Verification items for the finished model (mm, model axes). Round coordinates to 2 decimals unless told otherwise and drop trailing zeros. Order: outer loops, then holes, each group sorted by start corner. A loop starts at its lowest first (then second) coordinate and runs counter-clockwise, first axis right, second up. Notation, with made-up numbers: M 22.25,48.5 L 71.25,48.5 A36 ccw 71.25,84.5 Z; hole C -28.75,47.25 d7. An arc over 180 degrees is marked long. Use CSV: the item, a comma, the result in double quotes. Start each with the question number.
Q1. Gauge pin test, flat ends, axial feed: pin 1 Ø1.6 at (y, z) = (1, -34) entering from -X; pin 2 Ø1.1 at (y, z) = (2, -222) entering from +X; pin 3 Ø1 at (y, z) = (2, -64) entering from -X. Record the tip position at first contact, or that the pin passes through.
Q2. Sectioned sample at A-A (y = 0.75). State how many separate pieces and enclosed holes the cut face has, and give its area (3 significant figures).
Q3. Sectioned sample at B-B (z = -500). Enter the section's corners in (x, y).
Q4. Scan lines: line 1 (X direction, y = 0.95, z = -95); line 2 (X direction, y = 0.5, z = -28); line 3 (X direction, y = 1.1, z = -175). Record each from-to range of solid material in increasing order.
```python
from build123d import *

# Parameters (mm, degrees)
SALIENTE_EXTRUIR1_DEPTH = 3.2
CROQUIS3_R              = 2.05
CORTAR_EXTRUIR2_DEPTH   = 3.2
CORTAR_EXTRUIR3_DEPTH   = 3.2
CORTAR_EXTRUIR4_DEPTH   = 3.2
REDONDEO1_R             = 3
CROQUIS6_R              = 1.55
CORTAR_EXTRUIR5_DEPTH   = 3.2
CROQUIS7_W              = 3
CROQUIS7_H              = 0.2
CORTAR_EXTRUIR6_DEPTH   = 3.2


with BuildPart() as part:
    # Croquis1 → Saliente-Extruir1 (new body)
    with BuildSketch(Plane(origin=(0, 0, 0), x_dir=(1, 0, 0), z_dir=(0, 1, 0))):
        Polygon((7, 66.1), (10, 66.1), (10, 62.9), (7, 62.9), (7, 61.5), (3, 61.5), (3, 62.9), (0, 62.9), (0, 57), (-3, 57), (-3, 51), (0, 51), (0, 0), (165, 0), (165, 1.5), (168, 1.5), (168, 7.5), (165, 7.5), (165, 13.4), (162, 13.4), (162, 12), (158, 12), (158, 13.4), (155, 13.4), (155, 16.6), (158, 16.6), (158, 18), (162, 18), (162, 16.6), (165, 16.6), (165, 22.5), (168, 22.5), (168, 28.5), (165, 28.5), (165, 570), (30, 570), (30, 566.9), (21.6, 566.9), (21.6, 563.9), (23, 563.9), (23, 559.9), (21.6, 559.9), (21.6, 556.9), (18.4, 556.9), (18.4, 559.9), (17, 559.9), (17, 563.9), (18.4, 563.9), (18.4, 566.9), (10, 566.9), (10, 570), (0, 570), (0, 543), (-3, 543), (-3, 537), (0, 537), (0, 531.1), (3, 531.1), (3, 532.5), (7, 532.5), (7, 531.1), (10, 531.1), (10, 527.9), (7, 527.9), (7, 526.5), (3, 526.5), (3, 527.9), (0, 527.9), (0, 522), (-3, 522), (-3, 516), (0, 516), (0, 388), (-3, 388), (-3, 382), (0, 382), (0, 376.1), (3, 376.1), (3, 377.5), (7, 377.5), (7, 376.1), (10, 376.1), (10, 372.9), (7, 372.9), (7, 371.5), (3, 371.5), (3, 372.9), (0, 372.9), (0, 367), (-3, 367), (-3, 361), (0, 361), (0, 233), (-3, 233), (-3, 227), (0, 227), (0, 221.1), (3, 221.1), (3, 222.5), (7, 222.5), (7, 221.1), (10, 221.1), (10, 217.9), (7, 217.9), (7, 216.5), (3, 216.5), (3, 217.9), (0, 217.9), (0, 212), (-3, 212), (-3, 206), (0, 206), (0, 78), (-3, 78), (-3, 72), (0, 72), (0, 66.1), (3, 66.1), (3, 67.5), (7, 67.5), align=None)
    extrude(amount=SALIENTE_EXTRUIR1_DEPTH)

    # Croquis3 → Cortar-Extruir2 (cut)
    with BuildSketch(Plane(origin=(0, 3.2, 0), x_dir=(1, 0, 0), z_dir=(0, 1, 0))):
        with Locations((40, 80)):
            Circle(CROQUIS3_R)
        with Locations((90, 80)):
            Circle(CROQUIS3_R)
        with Locations((40, 230)):
            Circle(CROQUIS3_R)
    extrude(amount=-CORTAR_EXTRUIR2_DEPTH, mode=Mode.SUBTRACT)

    # Croquis4 → Cortar-Extruir3 (cut)
    with BuildSketch(Plane.XZ):
        with BuildLine():
            Line((143, -30.5), (129, -30.5))
            ThreePointArc((129, -30.5), (127.585786438, -31.085786438), (127, -32.5))
            Line((127, -32.5), (127, -38.5))
            ThreePointArc((127, -38.5), (127.585786438, -39.914213562), (129, -40.5))
            Line((129, -40.5), (143, -40.5))
            ThreePointArc((143, -40.5), (144.414213562, -39.914213562), (145, -38.5))
            Line((145, -38.5), (145, -32.5))
            ThreePointArc((145, -32.5), (144.414213562, -31.085786438), (143, -30.5))
        make_face()
    extrude(amount=-CORTAR_EXTRUIR3_DEPTH, mode=Mode.SUBTRACT)

    # Croquis5 → Cortar-Extruir4 (cut)
    with BuildSketch(Plane.XZ):
        with BuildLine():
            Line((35, -570), (165, -570))
            Line((165, -570), (165, -31.5))
            ThreePointArc((165, -31.5), (70.982951471, -293.744955787), (35, -570))
        make_face()
    extrude(amount=-CORTAR_EXTRUIR4_DEPTH, mode=Mode.SUBTRACT)

    # Redondeo1
    redondeo1_edges = [part.edges().sort_by_distance(p)[0] for p in [
        (35, 1.6, -570),
    ]]
    fillet(redondeo1_edges, radius=REDONDEO1_R)

    # Croquis6 → Cortar-Extruir5 (cut)
    with BuildSketch(Plane.XZ):
        with Locations((110, -95)):
            Circle(CROQUIS6_R)
        with Locations((35, -95)):
            Circle(CROQUIS6_R)
        with Locations((60, -175)):
            Circle(CROQUIS6_R)
        with Locations((15, -175)):
            Circle(CROQUIS6_R)
        with Locations((77, -35.5)):
            Circle(CROQUIS6_R)
        with Locations((37, -215.5)):
            Circle(CROQUIS6_R)
        with Locations((57, -155.5)):
            Circle(CROQUIS6_R)
    extrude(amount=-CORTAR_EXTRUIR5_DEPTH, mode=Mode.SUBTRACT)

    # Croquis7 → Cortar-Extruir6 (cut)
    with BuildSketch(Plane.XZ):
        with Locations((-1.5, -542.9)):
            Rectangle(CROQUIS7_W, CROQUIS7_H)
        with Locations((-1.5, -537.1)):
            Rectangle(CROQUIS7_W, CROQUIS7_H)
        with Locations((-1.5, -521.9)):
            Rectangle(CROQUIS7_W, CROQUIS7_H)
        with Locations((-1.5, -516.1)):
            Rectangle(CROQUIS7_W, CROQUIS7_H)
        with Locations((-1.5, -387.9)):
            Rectangle(CROQUIS7_W, CROQUIS7_H)
        with Locations((-1.5, -382.1)):
            Rectangle(CROQUIS7_W, CROQUIS7_H)
        with Locations((-1.5, -366.9)):
            Rectangle(CROQUIS7_W, CROQUIS7_H)
        with Locations((-1.5, -361.1)):
            Rectangle(CROQUIS7_W, CROQUIS7_H)
        with Locations((-1.5, -232.9)):
            Rectangle(CROQUIS7_W, CROQUIS7_H)
        with Locations((-1.5, -227.1)):
            Rectangle(CROQUIS7_W, CROQUIS7_H)
        with Locations((-1.5, -211.9)):
            Rectangle(CROQUIS7_W, CROQUIS7_H)
        with Locations((-1.5, -206.1)):
            Rectangle(CROQUIS7_W, CROQUIS7_H)
        with Locations((-1.5, -77.9)):
            Rectangle(CROQUIS7_W, CROQUIS7_H)
        with Locations((-1.5, -72.1)):
            Rectangle(CROQUIS7_W, CROQUIS7_H)
        with Locations((-1.5, -51.1)):
            Rectangle(CROQUIS7_W, CROQUIS7_H)
        with Locations((-1.5, -56.9)):
            Rectangle(CROQUIS7_W, CROQUIS7_H)
        with Locations((166.5, -28.4)):
            Rectangle(CROQUIS7_W, CROQUIS7_H)
        with Locations((166.5, -22.6)):
            Rectangle(CROQUIS7_W, CROQUIS7_H)
        with Locations((166.5, -7.4)):
            Rectangle(CROQUIS7_W, CROQUIS7_H)
        with Locations((166.5, -1.6)):
            Rectangle(CROQUIS7_W, CROQUIS7_H)
    extrude(amount=-CORTAR_EXTRUIR6_DEPTH, mode=Mode.SUBTRACT)


solid = part.part
```
Verdict:
1,pin 1,"stops at x = 0"
1,pin 2,"stops at x = 90.66"
1,pin 3,"stops at x = 10"
2,separate pieces,"1"
2,enclosed holes,"11"
2,area,"47,600 mm²"
3,outline,"M 0,0 L 38.44,0 L 38.44,3.2 L 0,3.2 Z"
4,line 1,"x = 0 to 33.45, 36.55 to 108.45, 111.55 to 136.28"
4,line 2,"x = 0 to 168"
4,line 3,"x = 0 to 13.45, 16.55 to 58.45, 61.55 to 105.71"
